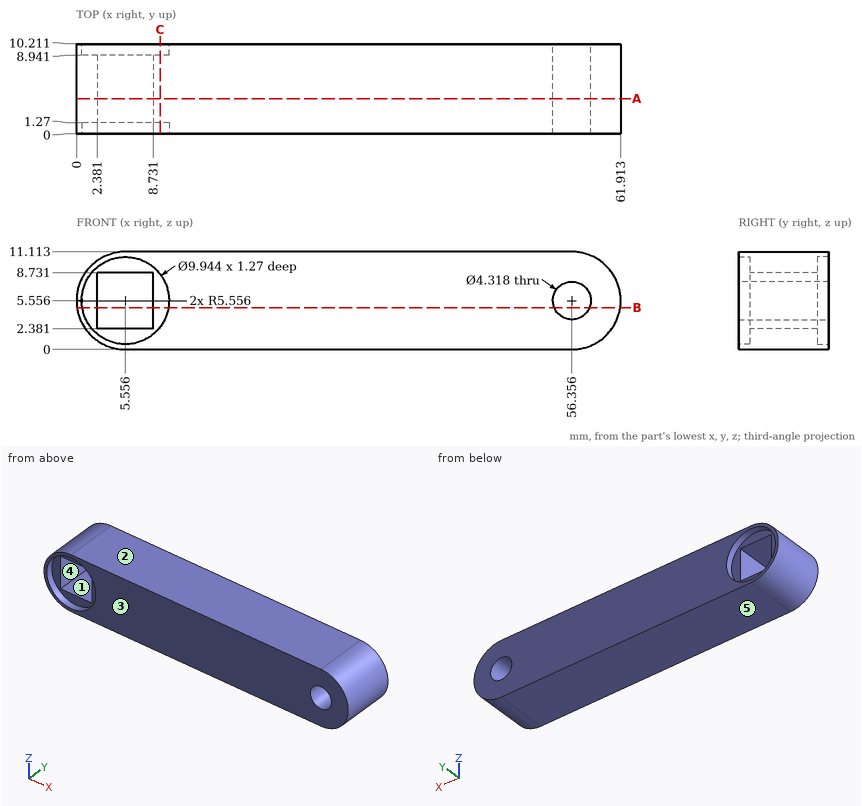
The drawing under review shows one solid part. Ordinate dimensions are in mm from its lowest x, y, z. A direction names the side the tool comes from. Round coordinates to 2 decimals unless told otherwise and drop trailing zeros. Write each loop counter-clockwise with the first axis right and the second up, starting at its lowest first coordinate (ties: lowest second). Pieces come first, ordered by that corner, then holes. Notation, with made-up numbers: (-34.75, -20.75) - (0.25, -20.75) arc R18 ccw to (0.25, -0.75) - close; hole circle Ø4 at (-5.75, 79.5). An arc over 180 degrees is marked (long way). Use a Markdown table: item, result. Add a question column.
1. For the marked faces 4 and 5, list the 3-axis set-ups (+Z, -Z, +X, -X, +Y, -Y) from which the entire face can be reached by the end or side of a thin tool; tool diameter is ignored.
2. Wall thickness on probe 1 along X at (y, z) = (4.75, 5.75) (1 decimal); probe 2 along X at (y, z) = (8.75, 7); probe 3 along Z at (x, y) = (55, 2) (1 decimal): over which ranges is each line inside the solid? List them lowest first.
3. Clearance check with flat-ended pins moving along their axes: pin 1 (5 mm diameter, centred on x = 6.5, z = 6.5, fed in from -Y); pin 2 (5 mm diameter, centred on y = 5.5, z = 2, fed in from -X). State where each tip first meets the part, or that it passes through.
4. We need section A-A (y = 4). State the section outline as (x, z) points (1 decimal).
5. We need section C-C (x = 9.5). State the section outline as (y, z) points (1 decimal).
6. Mouldability with a two-part tool opening along Z and no side actions: class the marked faces 1, 2 and 3 as +Z half, -Z half, draft (parallel to the pull), parting line (faces both ways), or undercut.
7. We need section B-B (z = 4.75). State the section outline as (x, y) points.
Output:
| question | item | result |
|---|---|---|
| 1 | face 4 | +Y, -Y |
| 1 | face 5 | -Z, +X, -X, +Y, -Y |
| 2 | probe 1 | x = 0 to 2.4, 8.7 to 54.2, 58.5 to 61.9 |
| 2 | probe 2 | x = 0.19 to 2.38, 8.73 to 54.75, 57.96 to 61.72 |
| 2 | probe 3 | z = 0 to 3.9, 7.2 to 11.1 |
| 3 | pin 1 | stops at y = 1.27 |
| 3 | pin 2 | stops at x = 0.1 |
| 4 | outline | (5.6, 0) - (56.4, 0) arc R5.6 ccw to (56.4, 11.1) - (5.6, 11.1) arc R5.6 ccw to start; hole (2.4, 2.4) - (8.7, 2.4) - (8.7, 8.7) - (2.4, 8.7) - close; hole circle Ø4.3 at (56.4, 5.6) |
| 5 | outline | (0, 0) - (10.2, 0) - (10.2, 2.5) - (8.9, 2.5) - (8.9, 8.6) - (10.2, 8.6) - (10.2, 11.1) - (0, 11.1) - (0, 8.6) - (1.3, 8.6) - (1.3, 2.5) - (0, 2.5) - close |
| 6 | face 1 | undercut |
| 6 | face 2 | +Z half |
| 6 | face 3 | draft |
| 7 | outline | (0.06, 0) - (0.65, 0) - (0.65, 1.27) - (2.38, 1.27) - (2.38, 8.94) - (0.65, 8.94) - (0.65, 10.21) - (0.06, 10.21) - close; (8.73, 1.27) - (10.46, 1.27) - (10.46, 0) - (54.35, 0) - (54.35, 10.21) - (10.46, 10.21) - (10.46, 8.94) - (8.73, 8.94) - close; (58.36, 0) - (61.85, 0) - (61.85, 10.21) - (58.36, 10.21) - close |
